Source: CAD feature listing. Evaluate the final solid. Frame: model axes, mm. Give positions to 0.01 mm unless a question says otherwise; leave off trailing zeros. Order: outer loops, then holes, each group sorted by start corner. A loop starts at its lowest first (then second) coordinate and runs counter-clockwise, first axis right, second up. Notation, with made-up numbers: (27, -28.75) -> (76, -28.75) arc R20 cw to (76, -7.75) -> close; hole circle Ø4 at (1, 67.25). An arc over 180 degrees is marked (long way). Answer in a Markdown table with one row per item.
```python
from build123d import *

# Parameters (mm, degrees)
F0_W     = 203.2
F0_H     = 152.4
F1_DEPTH = 3.175
F2_R     = 6.35
F3_DEPTH = 3.176
F4_W     = 203.2
F4_H     = 152.4
F4_W_2   = 127
F4_H_2   = 25.4
F5_DEPTH = 3.176
F6_R     = 6.35
F7_R     = 1.5875
F8_DEPTH = 3.176


with BuildPart() as f1:
    # F0 (on Top) → F1 (new body)
    with BuildSketch(Plane.XY):
        Rectangle(F0_W, F0_H)
    extrude(amount=F1_DEPTH)

    # F2 (on face) → F3 (cut, through all)
    with BuildSketch(Plane.XY.offset(3.175)):
        with Locations((-31.75, 0)):
            Circle(F2_R)
        with Locations((63.5, 0)):
            Circle(F2_R)
    extrude(amount=-F3_DEPTH, mode=Mode.SUBTRACT)

    # F4 (on face) → F5 (cut, through all)
    with BuildSketch(Plane.XY.offset(3.175)):
        Rectangle(F4_W, F4_H)
        with Locations((15.875, 0)):
            Rectangle(F4_W_2, F4_H_2, mode=Mode.SUBTRACT)
    extrude(amount=-F5_DEPTH, mode=Mode.SUBTRACT)

    # F6
    f6_edges = [f1.edges().sort_by_distance(p)[0] for p in [
        (-47.625, 12.7, 1.5875),
        (-47.625, -12.7, 1.5875),
        (79.375, -12.7, 1.5875),
        (79.375, 12.7, 1.5875),
    ]]
    fillet(f6_edges, radius=F6_R)

    # F7 (on face) → F8 (cut, through all)
    with BuildSketch(Plane.XY.offset(3.175)):
        Circle(F7_R)
        with Locations((31.75, 0)):
            Circle(F7_R)
    extrude(amount=-F8_DEPTH, mode=Mode.SUBTRACT)


solid = f1.part
```
(1) Ray query, probe 1 along Y at (x, z) = (0, 2.05); probe 2 along X at (y, z) = (-5, 0.3) (3 decimals); probe 3 along Y at (x, z) = (63.5, 0.8). Return the intervals inside material, ascending.
A:
| item | result |
|---|---|
| probe 1 | y = -12.7 to -1.59, 1.59 to 12.7 |
| probe 2 | x = -47.625 to -35.664, -27.836 to 59.586, 67.414 to 79.375 |
| probe 3 | y = -12.7 to -6.35, 6.35 to 12.7 |
(2) Pull-direction query (Y, two-part tool) for faces 1 (the flat face through (15, -12.7, 2)), 2 (the cylindrical face through (-0.34, -1.55, 1.61)), 3 (the cylindrical face through (-45.814, 10.79, 1.565)); classes: +Y half, -Y half, draft (parallel to the pull), parting line (faces both ways), or undercut.
A:
| item | result |
|---|---|
| face 1 | -Y half |
| face 2 | undercut |
| face 3 | +Y half |
(3) Section query D-D (x = 61). Return the cut outline in (y, z) (3 decimals), plus the area to 3 significant figures.
A:
| item | result |
|---|---|
| outline | (-12.7, 0) -> (-5.837, 0) -> (-5.837, 3.175) -> (-12.7, 3.175) -> close; (5.837, 0) -> (12.7, 0) -> (12.7, 3.175) -> (5.837, 3.175) -> close |
| area | 43.6 mm^2 |
(4) Section query C-C (x = 31.75). Return the cut outline in (y, z) (1 decimal), plus the area to 3 significant figures.
A:
| item | result |
|---|---|
| outline | (-12.7, 0) -> (-1.6, 0) -> (-1.6, 3.2) -> (-12.7, 3.2) -> close; (1.6, 0) -> (12.7, 0) -> (12.7, 3.2) -> (1.6, 3.2) -> close |
| area | 70.6 mm^2 |
(5) Section query A-A (y = 0). Give the number of separate pieces and of enclosed holes in the cut face, plus the area to 3 significant figures.
A:
| item | result |
|---|---|
| separate pieces | 5 |
| enclosed holes | 0 |
| area | 302 mm^2 |
